Check sheet for the modelled part. Datum: model origin and axes. Units: mm. Face numbers are marked on the shaded views. A direction names the side the tool comes from. Coordinates: 2 decimals unless noted, no trailing zeros. Loops run counter-clockwise (first coordinate to the right, second up) from the corner with the lowest first, then second, coordinate; pieces in that order, holes last.
```python
from build123d import *

# Parameters (mm, degrees)
F1_DEPTH = 55
F2_W     = 50
F2_H     = 14
F3_DEPTH = 5
F4_W     = 1
F4_H     = 12
F5_DEPTH = 112
F7_DEPTH = 110
F8_R     = 5


with BuildPart() as f1:
    # F0 (on Right) → F1 (new body, symmetric)
    with BuildSketch(Plane.YZ):
        with BuildLine():
            Line((29.25, -19.45), (29.25, 19.45))
            ThreePointArc((29.25, 19.45), (26.3796464556, 26.3796464556), (19.45, 29.25))
            Line((19.45, 29.25), (-19.45, 29.25))
            ThreePointArc((-19.45, 29.25), (-26.3796464556, 26.3796464556), (-29.25, 19.45))
            Line((-29.25, 19.45), (-29.25, -19.45))
            ThreePointArc((-29.25, -19.45), (-26.3796464556, -26.3796464556), (-19.45, -29.25))
            Line((-19.45, -29.25), (19.45, -29.25))
            ThreePointArc((19.45, -29.25), (26.3796464556, -26.3796464556), (29.25, -19.45))
        make_face()
        with BuildLine():
            ThreePointArc((17.45, 25.6500001997), (23.2482757469, 23.2482757469), (25.6500001997, 17.45))
            Line((25.6500001997, 17.45), (25.6500001997, -17.45))
            ThreePointArc((25.6500001997, -17.45), (23.2482757469, -23.2482757469), (17.45, -25.6500001997))
            Line((17.45, -25.6500001997), (-17.45, -25.6500001997))
            ThreePointArc((-17.45, -25.6500001997), (-23.2482757469, -23.2482757469), (-25.6500001997, -17.45))
            Line((-25.6500001997, -17.45), (-25.6500001997, 17.45))
            ThreePointArc((-25.6500001997, 17.45), (-23.2482757469, 23.2482757469), (-17.45, 25.6500001997))
            Line((-17.45, 25.6500001997), (17.45, 25.6500001997))
        make_face(mode=Mode.SUBTRACT)
    extrude(amount=F1_DEPTH, both=True)

    # F2 (on face) → F3 (cut)
    with BuildSketch(Plane.XZ.offset(29.25)):
        with Locations((0, -12.45)):
            Rectangle(F2_W, F2_H)
    extrude(amount=-F3_DEPTH, mode=Mode.SUBTRACT)

    # F4 (on face) → F5 (cut)
    with BuildSketch(Plane.YZ.offset(55)):
        with Locations((-26.1500001997, -11.45)):
            Rectangle(F4_W, F4_H)
    extrude(amount=-F5_DEPTH, mode=Mode.SUBTRACT)

    # F6 (on face) → F7 (join)
    with BuildSketch(Plane.YZ.offset(55)):
        with BuildLine():
            ThreePointArc((27.3493670633, -25.25), (23.8771887242, -28.1929971978), (19.45, -29.25))
            Line((19.45, -29.25), (70, -29.25))
            Line((70, -29.25), (84.7360996039, -29.3794282716))
            ThreePointArc((84.7360996039, -29.3794282716), (86.5921446829, -28.1669015856), (86.1891008154, -25.98683738))
            Line((86.1891008154, -25.98683738), (79.577611796, -19.1723148788))
            ThreePointArc((79.577611796, -19.1723148788), (78.278627167, -18.5696430639), (76.9096917505, -18.9898694416))
            Line((76.9096917505, -18.9898694416), (76.7505439798, -19.1143983305))
            ThreePointArc((76.7505439798, -19.1143983305), (75.997756862, -20.4472363949), (76.4079148199, -21.9219961042))
            Line((76.4079148199, -21.9219961042), (79.4891255871, -25.8597797712))
            Line((79.4891255871, -25.8597797712), (71.1479993126, -25.8597797712))
            ThreePointArc((71.1479993126, -25.8597797712), (67.7312883661, -25.0716330431), (65.0050567922, -22.8664685681))
            Line((65.0050567922, -22.8664685681), (27.1680559872, 25.4891731038))
            ThreePointArc((27.1680559872, 25.4891731038), (28.7149055223, 22.6439827273), (29.25, 19.45))
            Line((29.25, 19.45), (29.25, 16.3374962926))
            Line((29.25, 16.3374962926), (51.9267094517, -12.6433112031))
            ThreePointArc((51.9267094517, -12.6433112031), (52.7956202032, -20.8667109465), (45.7837669312, -25.25))
            Line((45.7837669312, -25.25), (27.3493670633, -25.25))
        make_face()
    extrude(amount=-F7_DEPTH)

    # F8
    f8_edges = [f1.edges().sort_by_distance(p)[0] for p in [
        (-25, -27.95, -5.45),
        (-25, -27.326179, -19.45),
        (25, -27.326179, -19.45),
        (25, -27.95, -5.45),
    ]]
    fillet(f8_edges, radius=F8_R)


solid = f1.part
```
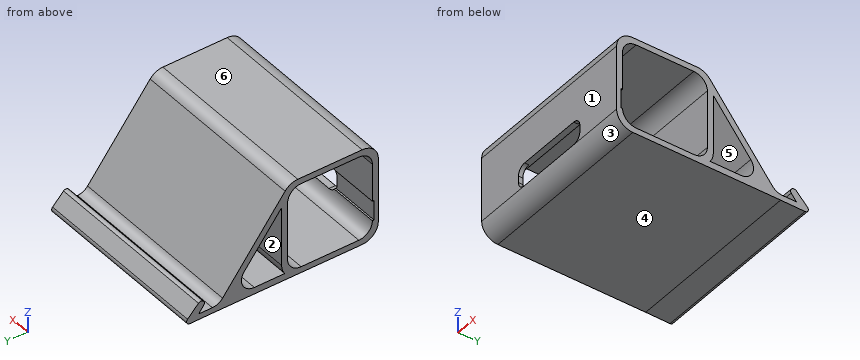
1) Depth check by flat-ended pin: pin 1 (12 mm diameter, centred on x = 2, y = 30.5, fed in from +Z); pin 2 (1.1 mm diameter, centred on x = -5.5, y = -27, fed in from -Z); pin 3 (17.5 mm diameter, centred on x = 26.5, y = 7.5, fed in from -Z). Enter the tip coordinate at first touch or a pass-through.
Answer sheet:
pin 1: stops at z = 27.85
pin 2: stops at z = -26.31
pin 3: stops at z = -29.25
2) Mould release check, pull along Z, two halves, no side actions. Record for the marked faces 1, 2 and 3: +Z half, -Z half, draft (parallel to the pull), parting line (faces both ways), or undercut.
Answer sheet:
face 1: draft
face 2: undercut
face 3: -Z half
3) Section check B-B on x = 35. Give the number of separate pieces and of enclosed holes in the cut face, plus the area to 3 significant figures.
Answer sheet:
separate pieces: 1
enclosed holes: 2
area: 1,320 mm2
4) Section check D-D on z = 4.5. Enter the section's corners in (x, y), plus the area to 3 significant figures.
Answer sheet:
outline: (-55, -29.25) - (55, -29.25) - (55, -25.65) - (-55, -25.65) - close; (-55, 25.65) - (55, 25.65) - (55, 29.25) - (-55, 29.25) - close; (-55, 38.51) - (55, 38.51) - (55, 43.59) - (-55, 43.59) - close
area: 1,350 mm2
5) Scan lines: line 1 (Z direction, x = 33, y = -5.5); line 2 (Z direction, x = 42, y = 18); line 3 (Y direction, x = -19, z = 6.5). Record each from-to range of solid material in increasing order.
Answer sheet:
line 1: z = -29.25 to -25.65, 25.65 to 29.25
line 2: z = -29.25 to -25.63, 25.63 to 29.25
line 3: y = -29.25 to -25.65, 25.65 to 29.25, 36.95 to 42.03
6) Section check A-A on y = 6. Enter the section's corners in (x, z).
Answer sheet:
outline: (-55, -29.25) - (55, -29.25) - (55, -25.65) - (-55, -25.65) - close; (-55, 25.65) - (55, 25.65) - (55, 29.25) - (-55, 29.25) - close
7) Set-up check for the marked faces 4, 5 and 6: record each of +Z, -Z, +X, -X, +Y, -Y from which the full face is reachable in a straight line by a thin tool's end or side.
Answer sheet:
face 4: -Z, +X, -X, -Y
face 5: +X, -X
face 6: +Z, +X, -X, +Y, -Y
